Design review of the part built by this model. Coordinates are the model's own, in mm. Face numbers are marked on the shaded views. A direction names the side the tool comes from. Round coordinates to 2 decimals unless told otherwise and drop trailing zeros. Order: outer loops, then holes, each group sorted by start corner. A loop starts at its lowest first (then second) coordinate and runs counter-clockwise, first axis right, second up. Notation, with made-up numbers: (24, -17.5) - (70, -17.5) arc R10 ccw to (70, -4.5) - close; hole circle Ø8 at (-4, -34). An arc over 180 degrees is marked (long way). Write item = value, one per line.
from build123d import *

# Parameters (mm, degrees)
F0_R     = 3.6
F1_DEPTH = 15
F0_R_2   = 7.5
F2_DEPTH = 5
F3_R     = 1


with BuildPart() as f1:
    # F0 (on Top) → F1 (new body)
    with BuildSketch(Plane.XY):
        Circle(F0_R)
    extrude(amount=F1_DEPTH)

    # F0 (on Top) → F2 (join)
    with BuildSketch(Plane.XY):
        Circle(F0_R_2)
        Circle(F0_R, mode=Mode.SUBTRACT)
        Circle(F0_R)
    extrude(amount=-F2_DEPTH)

    # F3
    f3_edges = [f1.edges().sort_by_distance(p)[0] for p in [
        (-3.6, 0, 15),
        (-7.5, 0, -5),
    ]]
    fillet(f3_edges, radius=F3_R)


solid = f1.part
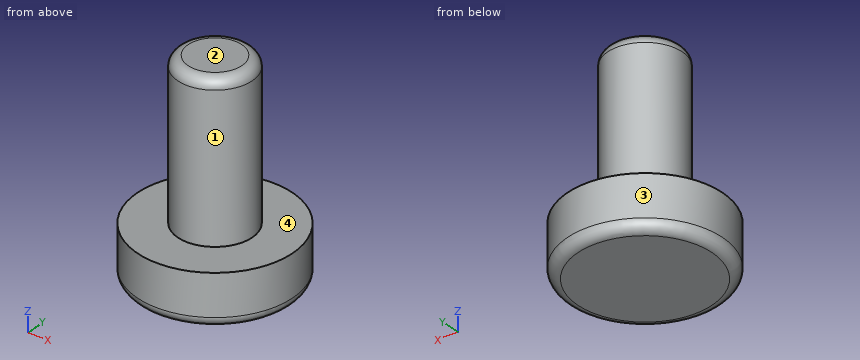
1) We need section C-C on z = 8.25. Write out the cut boundary in (x, y).
Findings:
outline = circle Ø7.2 at (0, 0)
2) To check wall thickness, follow L1, parallel to Z at x = -5, y = 2.5; L2, parallel to Y at x = -2.5, z = 12.25; L3, parallel to Z at x = 6.5, y = -2.5. State the ranges of each line that lie inside material, in increasing order. Write a range as from..to.
Findings:
L1 = -5..0
L2 = -2.59..2.59
L3 = -4.89..0
3) We need section D-D on z = -3.25. Write out the cut boundary in (x, y), and give its area (3 significant figures).
Findings:
outline = circle Ø15 at (0, 0)
area = 177 mm^2
4) For the marked faces 3 and 4, list the 3-axis set-ups (+Z, -Z, +X, -X, +Y, -Y) from which the entire face can be reached by the end or side of a thin tool; tool diameter is ignored.
Findings:
face_3 = +Z, -Z
face_4 = +Z
5) The part is to be moulded in two halves that separate along X. For the marked faces 1 and 2, say which applies: released by +X, released by -X, zero draft, split by the parting line, or undercut.
Findings:
face_1 = split by the parting line
face_2 = zero draft
6) We need section A-A on x = 0. Write out the cut boundary in (y, z), and give its area (3 significant figures).
Findings:
outline = (-7.5, -4) arc R1 ccw to (-6.5, -5) - (6.5, -5) arc R1 ccw to (7.5, -4) - (7.5, 0) - (3.6, 0) - (3.6, 14) arc R1 ccw to (2.6, 15) - (-2.6, 15) arc R1 ccw to (-3.6, 14) - (-3.6, 0) - (-7.5, 0) - close
area = 182 mm^2
7) Clearance check with flat-ended pins moving along their axes: pin 1 Ø4 at (y, z) = (-1, 8) entering from -X; pin 2 Ø1 at (y, z) = (-2, 2.5) entering from -X; pin 3 Ø5 at (y, z) = (-1, 12.5) entering from +X. State where each tip first meets the part, or that it passes through.
Findings:
pin_1 = -3.6
pin_2 = -3.27
pin_3 = 3.6
